Autodesk Inventor part; units mm, degrees
ref_plane "YZ Plane" through (0, 0, 0) normal (1, 0, 0) x (0, 1, 0)
ref_plane "XZ Plane" through (0, 0, 0) normal (0, 1, 0) x (-1, 0, 0)
ref_plane "XY Plane" through (0, 0, 0) normal (0, 0, 1) x (1, 0, 0)
sketch "Szkic1" plane through (0, 0, 0) normal (0, 1, 0) x (-1, 0, 0)
  line L0 (-10.5, -21.75) -> (10.5, -21.75)
  line L1 (10.5, -21.75) -> (10.5, 21.75)
  line L2 (10.5, 21.75) -> (-10.5, 21.75)
  line L3 (-10.5, 21.75) -> (-10.5, -21.75)
  line L4 (-10.5, -21.75) -> (10.5, 21.75) construction
  line L5 (10.5, -21.75) -> (-10.5, 21.75) construction
  point P0 (0, 0)
  dimension "d0" = 21
  dimension "d1" = 43.5
extrude "Wyciągnięcie proste1" add sketch "Szkic1" along normal blind 2
sketch "Szkic2" plane through (0, 2, 0) normal (0, 1, 0) x (1, 0, 0)
  line L0 (10.5, 21.75) -> (-10.5, 21.75)
  line L1 (-10.5, 21.75) -> (-10.5, -21.75)
  line L2 (-10.5, -21.75) -> (10.5, -21.75)
  line L3 (10.5, -21.75) -> (10.5, 21.75)
  point P0 (0, 0)
  point P1 (-7.5, -14.75)
  point P2 (7.5, 15.25)
  dimension "d4" = 3
  dimension "d5" = 7
  dimension "d6" = 6.5
  dimension "d7" = 3
hole "Otwór1" at (-7.5, 2, 14.75) at (7.5, 2, -15.25) direction (0, -1, 0) diameter 3 end through all
sketch "Szkic3" plane through (0, 2, 0) normal (0, 1, 0) x (1, 0, 0)
  line L0 (-7.1772, -9.2041) -> (7.109, -9.2041)
  line L1 (7.109, -9.2041) -> (7.109, -0.6113)
  line L2 (-7.1772, -9.2041) -> (-7.1772, -0.6113)
  line L3 (-7.1772, -0.6113) -> (7.109, -0.6113)
  line L4 (10.3774, 10.4592) -> (3.208, 10.4592)
  line L5 (3.208, 10.4592) -> (3.208, 2.868)
  line L6 (3.208, 2.868) -> (10.3774, 2.868)
  line L7 (10.3774, 2.868) -> (10.3774, 10.4592)
  line L8 (10.3774, 10.4592) -> (3.208, 2.868) construction
  line L9 (3.208, 10.4592) -> (10.3774, 2.868) construction
  line L10 (-5.7011, 15.0455) -> (-8.6533, 15.0455)
  line L11 (-8.6533, 15.0455) -> (-8.6533, 4.924)
  line L12 (-8.6533, 4.924) -> (-5.7011, 4.924)
  line L13 (-5.7011, 4.924) -> (-5.7011, 15.0455)
  line L14 (-5.7011, 15.0455) -> (-8.6533, 4.924) construction
  line L15 (-8.6533, 15.0455) -> (-5.7011, 4.924) construction
  circle A0 centre (0.6572, -16.8759) radius 3.3835
  circle A1 centre (1.2574, 17.1015) radius 3.1458
  point P0 (0, 0)
  point P1 (6.7927, 6.6636)
  point P2 (-7.1772, 9.9848)
extrude "Wyciągnięcie proste2" add sketch "Szkic3" along normal blind 10
properties part number "step up"
Verification items for the finished model (mm, model axes). A direction names the side the tool comes from. Round coordinates to 2 decimals unless told otherwise and drop trailing zeros. Loops run counter-clockwise (first coordinate to the right, second up) from the corner with the lowest first, then second, coordinate; pieces in that order, holes last. Notation, with made-up numbers: (61, 42) -> (67, 42) arc R21 ccw to (67, 63) -> close; hole circle Ø4 at (61.5, 30). An arc over 180 degrees is marked (long way). Answer as a JSON object with one key per item and string values.
Q1. Section check B-B (z = 15). Record the boundary of the cut face in (x, y), then the cut area to 3 significant figures.
Data:
{"outline": "(-10.5, 0) -> (-8.98, 0) -> (-8.98, 2) -> (-10.5, 2) -> close; (-6.02, 0) -> (10.5, 0) -> (10.5, 2) -> (3.47, 2) -> (3.47, 12) -> (-2.16, 12) -> (-2.16, 2) -> (-6.02, 2) -> close", "area": "92.4 mm2"}
Q2. Draft check along X on faces 1 (the flat face through (7.109, 7, 5)), 2 (the flat face through (-7, 7, -4.924)), 3 (the cylindrical face through (-6.59, 0.99, 13.56)). Enter one of: pulls with the +X half, pulls with the -X half, needs draft (parallel to the pull), parting line crosses it, or undercut.
Data:
{"face 1": "pulls with the +X half", "face 2": "needs draft", "face 3": "undercut"}
Q3. Section check D-D (y = 1.5). Record the boundary of the cut face in (x, z).
Data:
{"outline": "(-10.5, -21.75) -> (10.5, -21.75) -> (10.5, 21.75) -> (-10.5, 21.75) -> close; hole circle Ø3 at (-7.5, 14.75); hole circle Ø3 at (7.5, -15.25)"}
Q4. Access from +Z, -Z, +X, -X, +Y, -Y to the whole of each face (thin tool, end or side, straight path). Record for faces 4 (the flat face through (0, 7, 9.204)), 5 (the flat face through (3.208, 7, -7)), 6 (the flat face through (-7.177, 7, 5)).
Data:
{"face 4": "+X, -X, +Y", "face 5": "+Y", "face 6": "+Z, -X, +Y"}
Q5. Section check A-A (x = -6.75). Record the boundary of the cut face in (y, z), then the cut area to 3 significant figures.
Data:
{"outline": "(0, -21.75) -> (2, -21.75) -> (2, -15.05) -> (12, -15.05) -> (12, -4.92) -> (2, -4.92) -> (2, 0.61) -> (12, 0.61) -> (12, 9.2) -> (2, 9.2) -> (2, 13.45) -> (0, 13.45) -> close; (0, 16.05) -> (2, 16.05) -> (2, 21.75) -> (0, 21.75) -> close", "area": "269 mm2"}
Q6. Scan lines: line 1 (Z direction, x = 7.5, y = 0.6); line 2 (X direction, y = 1.5, z = -15.25); line 3 (Z direction, x = 3.75, y = 8.5). Record each from-to range of solid material in increasing order. Write a range as from..to.
Data:
{"line 1": "z = -21.75..-16.75, -13.75..21.75", "line 2": "x = -10.5..6, 9..10.5", "line 3": "z = -19.02..-15.18, -10.46..-2.87, 0.61..9.2, 15.5..18.25"}
Q7. Go/stop test with flat-tipped pins: P1, Ø5, axis at x = 7.5, z = -15.25, coming from the -Y side; P2, Ø7, axis at y = 7, z = 6, coming from the -X side; P3, Ø5.5, axis at x = 5.5, y = 7, coming from the -Z side; P4, Ø6, axis at x = -2, y = 9.5, coming from the -Z side. Record where each tip stops, or that it passes through.
Data:
{"P1": "stops at y = 0", "P2": "stops at x = -7.18", "P3": "stops at z = -19.87", "P4": "stops at z = -20.24"}
Q8. Section check C-C (y = 4.75). Record the boundary of the cut face in (x, z), then the cut area to 3 significant figures.
Data:
{"outline": "(-8.65, -15.05) -> (-5.7, -15.05) -> (-5.7, -4.92) -> (-8.65, -4.92) -> close; (-7.18, 0.61) -> (7.11, 0.61) -> (7.11, 9.2) -> (-7.18, 9.2) -> close; circle Ø6.77 at (0.66, 16.88); circle Ø6.29 at (1.26, -17.1); (3.21, -10.46) -> (10.38, -10.46) -> (10.38, -2.87) -> (3.21, -2.87) -> close", "area": "274 mm2"}
